The listing builds one solid part. Answer for the finished solid, in the listing's coordinates (mm). A direction names the side the tool comes from. Give positions to 0.01 mm unless a question says otherwise; leave off trailing zeros. Loops run counter-clockwise (first coordinate to the right, second up) from the corner with the lowest first, then second, coordinate; pieces in that order, holes last. Notation, with made-up numbers: M 2,-24.75 L 6,-24.75 A10 ccw 6,-17.75 Z; hole C -31,-21 d3. An arc over 180 degrees is marked long. Return JSON: item names as keys, results as strings.
from build123d import *

# Parameters (mm, degrees)
BOSS_EXTRUDE1_DEPTH = 9
CUT_EXTRUDE1_DEPTH  = 25
BOSS_EXTRUDE2_DEPTH = 18
LPATTERN1_COUNT     = 5
LPATTERN1_PITCH     = 5
FILLET1_R           = 6
FILLET2_R           = 5
SKETCH4_R           = 1.5
CUT_EXTRUDE2_DEPTH  = 25
SKETCH5_R           = 1.5
CUT_EXTRUDE3_DEPTH  = 25
CUT_EXTRUDE4_DEPTH  = 2
CUT_EXTRUDE5_DEPTH  = 2


with BuildPart() as part:
    # Sketch1 → Boss-Extrude1 (new, symmetric)
    with BuildSketch(Plane(origin=(0, 0, 0), x_dir=(0, 0, -1), z_dir=(1, 0, 0))):
        Polygon((72.723807427, -0.926412344), (62.92004934, -2.897789372), (49.12041015, 65.728517233), (72.723807427, 70.073587656), align=None)
        Polygon((91.582675421, -7.328280768), (98.60593402, -0.20972483), (90.120652646, 8.275556545), (79.096697455, -2.897980722), (72.723807427, -0.926412344), (62.92004934, -2.897789372), (58.018170297, -3.883477885), (58.018170297, -13.883477885), (66.142055029, -24.032492461), (80.582675421, -50.328280768), (80.582675421, -57.328280768), (91.582675421, -57.328280768), align=None)
        with BuildLine():
            ThreePointArc((98.60593402, -0.20972483), (98.60593402, 8.275556545), (90.120652646, 8.275556545))
            Line((90.120652646, 8.275556545), (98.60593402, -0.20972483))
        make_face()
    extrude(amount=BOSS_EXTRUDE1_DEPTH, both=True)

    # Sketch2 → Cut-Extrude1 (cut)
    with BuildSketch(Plane(origin=(9, 0, 0), x_dir=(0, 0, -1), z_dir=(1, 0, 0))):
        Polygon((88.882675421, -50.328280768), (88.882675421, -25.328280768), (73.882675421, -25.328280768), align=None)
    extrude(amount=-CUT_EXTRUDE1_DEPTH, mode=Mode.SUBTRACT)

    # Sketch3 → Boss-Extrude2 (add)
    with BuildSketch(Plane(origin=(9, 0, 0), x_dir=(0, 0, -1), z_dir=(1, 0, 0))):
        Polygon((91.582675421, -50.328280768), (91.582675421, -52.328280768), (95.582675421, -50.328280768), align=None)
        Polygon((91.582675421, -50.328280768), (95.582675421, -50.328280768), (91.582675421, -48.328280768), align=None)
    boss_extrude2 = extrude(amount=-BOSS_EXTRUDE2_DEPTH)

    # LPattern1: Boss-Extrude2 ×5
    with Locations(*[(0, i * LPATTERN1_PITCH, 0) for i in range(1, LPATTERN1_COUNT)]):
        add(boss_extrude2)

    # Fillet1
    fillet1_edges = [part.edges().sort_by_distance(p)[0] for p in [
        (0, -13.883477885, -58.018170297),
        (0, -3.883477885, -58.018170297),
    ]]
    fillet(fillet1_edges, radius=FILLET1_R)

    # Fillet2
    fillet2_edges = [part.edges().sort_by_distance(p)[0] for p in [
        (0, 65.728517233, -49.12041015),
        (0, 70.073587656, -72.723807427),
    ]]
    fillet(fillet2_edges, radius=FILLET2_R)

    # Sketch4 → Cut-Extrude2 (cut)
    with BuildSketch(Plane(origin=(9, 0, 0), x_dir=(0, 0, -1), z_dir=(1, 0, 0))):
        with Locations((55.024265961, 61.731324387)):
            Circle(SKETCH4_R)
    extrude(amount=-CUT_EXTRUDE2_DEPTH, mode=Mode.SUBTRACT)

    # Sketch5 → Cut-Extrude3 (cut)
    with BuildSketch(Plane(origin=(9, 0, 0), x_dir=(0, 0, -1), z_dir=(1, 0, 0))):
        with Locations((94.363293333, 4.032915857)):
            Circle(SKETCH5_R)
        with Locations((64.018170297, -8.79707708)):
            Circle(SKETCH5_R)
    extrude(amount=-CUT_EXTRUDE3_DEPTH, mode=Mode.SUBTRACT)

    # Sketch6 → Cut-Extrude4 (cut)
    with BuildSketch(Plane(origin=(9, 0, 0), x_dir=(0, 0, -1), z_dir=(1, 0, 0))):
        with BuildLine():
            Line((68.990160428, 15.050217447), (68.990160428, 49.050217447))
            Line((68.990160428, 49.050217447), (58.046044594, 47.035551784))
            Line((58.046044594, 47.035551784), (64.354451081, 15.663525908))
            ThreePointArc((64.354451081, 15.663525908), (66.453192239, 13.700695979), (68.990160428, 15.050217447))
        make_face()
    extrude(amount=-CUT_EXTRUDE4_DEPTH, mode=Mode.SUBTRACT)

    # Sketch7 → Cut-Extrude5 (cut)
    with BuildSketch(Plane.ZY.offset(9)):
        with BuildLine():
            Line((-68.307430595, 48.924535996), (-56.93452281, 46.830935459))
            Line((-56.93452281, 46.830935459), (-63.369204726, 14.830935459))
            ThreePointArc((-63.369204726, 14.830935459), (-65.88423927, 12.454979569), (-68.307430595, 14.924535996))
            Line((-68.307430595, 14.924535996), (-68.307430595, 48.924535996))
        make_face()
    extrude(amount=-CUT_EXTRUDE5_DEPTH, mode=Mode.SUBTRACT)


solid = part.part
(1) A tool of negligible diameter and unlimited length cuts with its end or side. For faces 1 (the flat face through (0.126, -37.653, -81.278)), 2 (the flat face through (0.13, 2.77, -84.69)), 3 (the flat face through (7, 36, -65)), 4 (the flat face through (0, -54, -80.583)), 5 (the flat face through (0.126, -46.342, -93.555)), from which of +Z, -Z, +X, -X, +Y, -Y can it reach the whole face along a straight path? Write none if from no direction.
Values follow:
{"face 1": "+X, -X", "face 2": "+X, -X, +Y", "face 3": "+X", "face 4": "+Z, +X, -X, -Y", "face 5": "-Z, +X, -X"}
(2) The part is cut by section B-B (y = 23.5). Determine the outline of the cut face in (x, z), and give its area (3 significant figures).
Values follow:
{"outline": "M -9,-72.72 L 9,-72.72 L 9,-68.99 L 7,-68.99 L 7,-62.78 L 9,-62.78 L 9,-57.61 L -9,-57.61 L -9,-61.63 L -7,-61.63 L -7,-68.31 L -9,-68.31 Z", "area": "246 mm²"}
(3) Determine the mould class of faces 6 (the flat face through (0.13, -29.34, -93.61)), 7 (the flat face through (0, -57.328, -86)), 8 (the cylindrical face through (0.126, 62.745, -53.919)) for opening direction Z: released by +Z, released by -Z, zero draft, split by the parting line, or undercut.
Values follow:
{"face 6": "released by -Z", "face 7": "zero draft", "face 8": "undercut"}
(4) Given pin 1 (2 mm diameter, centred on x = 1, z = -62, fed in from +Y); pin 2 (3 mm diameter, centred on y = -14.5, z = -58.5, fed in from +X); pin 3 (10 mm diameter, centred on x = 7, y = -22, fed in from +Z); pin 4 (0.5 mm diameter, centred on x = -1, y = -33, fed in from -Z), each flat-ended and moving along its own axis, determine where each tip first touches the part or whether it passes through.
Values follow:
{"pin 1": "y = 68.28", "pin 2": "x = 9", "pin 3": "z = -60.51", "pin 4": "z = -91.58"}
(5) The part is cut by section C-C (z = -87.5). Determine the outline of the cut face in (x, y), and give its area (3 significant figures).
Values follow:
{"outline": "M -9,-57.33 L 9,-57.33 L 9,-48.02 L -9,-48.02 Z; M -9,-25.33 L 9,-25.33 L 9,5.62 L -9,5.62 Z", "area": "725 mm²"}
(6) Straight lines are drawn through the part: line 1 along Y through (x, z) = (-5.5, -86); line 2 along Z through (x, y) = (3.5, -39.5); line 3 along Y through (x, z) = (5.5, -92). For each, find the intervals that lie inside material, in ascending order.
Values follow:
{"line 1": "-57.33 to -45.52, -25.33 to 4.1", "line 2": "-93.93 to -88.88, -82.39 to -74.64", "line 3": "-52.12 to -48.54, -47.12 to -43.54, -42.12 to -38.54, -37.12 to -33.54, -32.12 to -28.54, -6.91 to 9.55"}
(7) The part is cut by section D-D (x = 5). Give the number of separate pieces and of enclosed holes in the cut face, and give its area (3 significant figures).
Values follow:
{"separate pieces": "1", "enclosed holes": "4", "area": "2,420 mm²"}
(8) The part is cut by section A-A (z = -60.5). Determine the outline of the cut face in (x, y).
Values follow:
{"outline": "M -9,-16.98 L 9,-16.98 L 9,-3.94 L -9,-3.94 Z; M -9,9.14 L 9,9.14 L 9,34.83 L 7,34.83 L 7,47.49 L 9,47.49 L 9,67.82 L -9,67.82 L -9,47.49 L -7,47.49 L -7,29.1 L -9,29.1 Z"}
